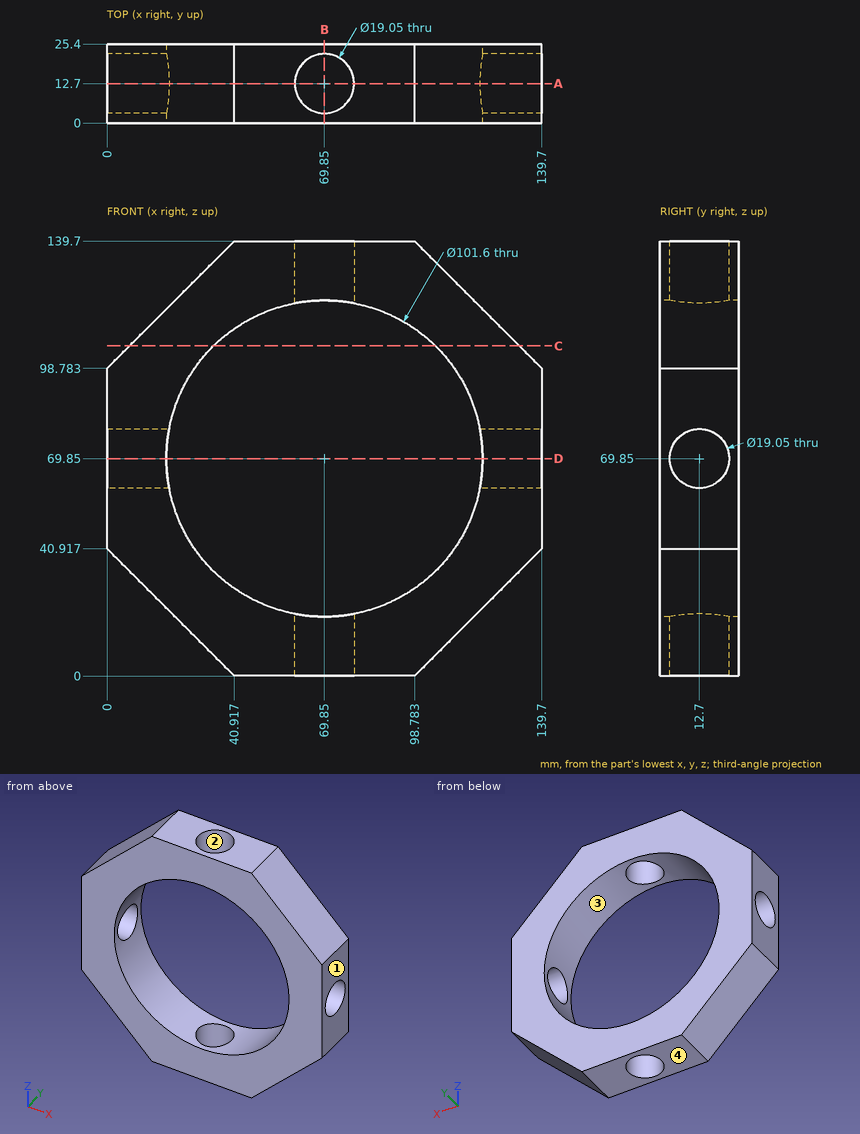
Study the drawing (mm; zero at the part's minimum x, y, z) and answer. Give positions to 0.01 mm unless a question says otherwise; leave off trailing zeros. Order: outer loops, then holes, each group sorted by start corner. A loop starts at its lowest first (then second) coordinate and runs counter-clockwise, first axis right, second up. Notation, with made-up numbers: (57, 62) -> (70, 62) arc R17 cw to (70, 67) -> close; hole circle Ø2 at (45.5, 35). An arc over 180 degrees is marked (long way). Put each result on its own line as item: value.
Item 1: A cutting plane is placed at D-D on z = 69.85. Give the vertices of the cut face in (x, y) (3 decimals), plus the area to 3 significant figures.
Established:
outline: (0, 0) -> (19.05, 0) -> (19.05, 3.175) -> (0, 3.175) -> close; (0, 22.225) -> (19.05, 22.225) -> (19.05, 25.4) -> (0, 25.4) -> close; (120.65, 0) -> (139.7, 0) -> (139.7, 3.175) -> (120.65, 3.175) -> close; (120.65, 22.225) -> (139.7, 22.225) -> (139.7, 25.4) -> (120.65, 25.4) -> close
area: 242 mm^2
Item 2: A cutting plane is placed at B-B on x = 69.85. Give the vertices of the cut face in (y, z) (3 decimals), plus the area to 3 significant figures.
Established:
outline: (0, 0) -> (3.175, 0) -> (3.175, 19.05) -> (0, 19.05) -> close; (0, 120.65) -> (3.175, 120.65) -> (3.175, 139.7) -> (0, 139.7) -> close; (22.225, 0) -> (25.4, 0) -> (25.4, 19.05) -> (22.225, 19.05) -> close; (22.225, 120.65) -> (25.4, 120.65) -> (25.4, 139.7) -> (22.225, 139.7) -> close
area: 242 mm^2
Item 3: For a pull along X with two mould halves and no side action, classify the marked faces 1, 2, 3 and 4 as released by +X, released by -X, zero draft, split by the parting line, or undercut.
Established:
face 1: released by +X
face 2: undercut
face 3: undercut
face 4: zero draft
Item 4: Given P1, Ø1.5, axis at x = 16, y = 9, coming from the -Z side; P2, Ø4, axis at x = 107, y = 6, coming from the +Z side; P3, Ø6, axis at x = 29.5, y = 2.5, coming from the +Z side, each flat-ended and moving along its own axis, determine where each tip first touches the part or whether it passes through.
Established:
P1: stops at z = 24.17
P2: stops at z = 133.48
P3: stops at z = 131.28
Item 5: A cutting plane is placed at A-A on y = 12.7. Count the separate pieces of the cut face and the enclosed holes in it, plus the area to 3 significant figures.
Established:
separate pieces: 4
enclosed holes: 0
area: 6,590 mm^2
Item 6: Straight lines are drawn through the part: line 1 (Y direction, x = 69, z = 4); line 2 (Z direction, x = 107.5, y = 7.5) (1 decimal); line 3 (X direction, y = 7, z = 98). For each, find the intervals that lie inside material, in ascending order.
Established:
line 1: y = 0 to 3.21, 22.19 to 25.4
line 2: z = 8.7 to 35.7, 104 to 131
line 3: x = 0 to 27.56, 112.14 to 139.7
Item 7: A cutting plane is placed at C-C on z = 106. Give the vertices of the cut face in (x, y), plus the area to 3 significant figures.
Established:
outline: (7.22, 0) -> (34.16, 0) -> (34.16, 25.4) -> (7.22, 25.4) -> close; (105.54, 0) -> (132.48, 0) -> (132.48, 25.4) -> (105.54, 25.4) -> close
area: 1,370 mm^2
